```python
from build123d import *

# Parameters (mm, degrees)
BOSS_EXTRUDE1_DEPTH = 4
SKETCH7_R           = 2
CUT_EXTRUDE1_DEPTH  = 4


with BuildPart() as part:
    # Sketch1 → Boss-Extrude1 (new body)
    with BuildSketch(Plane(origin=(0, 0, 0), x_dir=(1, 0, 0), z_dir=(0, 1, 0))):
        Polygon((-125, 115), (-125, 65), (-85, 41.905989232), (-85, -41.905989232), (-125, -65), (-125, -115), (-115, -125), (-65, -125), (-41.905989232, -85), (41.905989232, -85), (65, -125), (115, -125), (125, -115), (125, -65), (85, -41.905989232), (85, 41.905989232), (125, 65), (125, 115), (115, 125), (65, 125), (41.905989232, 85), (-41.905989232, 85), (-65, 125), (-115, 125), align=None)
    extrude(amount=BOSS_EXTRUDE1_DEPTH)

    # Sketch7 → Cut-Extrude1 (cut)
    with BuildSketch(Plane.XZ):
        with Locations(Location((96.392180149, -96.396634108, 0), (0, 0, 270))):
            Circle(SKETCH7_R)
        with Locations(Location((-96.396634108, -96.392180149, 0), (0, 0, 270))):
            Circle(SKETCH7_R)
        with Locations(Location((-96.392180149, 96.396634108, 0), (0, 0, 270))):
            Circle(SKETCH7_R)
        with Locations(Location((96.396634108, 96.392180149, 0), (0, 0, 270))):
            Circle(SKETCH7_R)
        with BuildLine():
            Line((112.617319154, -91.199448609), (97.141666667, -78.666998145))
            Line((97.141666667, -78.666998145), (95.253658711, -80.998398145))
            Line((95.253658711, -80.998398145), (110.729311198, -93.530848609))
            ThreePointArc((110.729311198, -93.530848609), (111.462995743, -94.910428371), (110.980579079, -96.396634108))
            ThreePointArc((110.980579079, -96.396634108), (103.942611055, -103.946782572), (96.392180149, -110.984447587))
            ThreePointArc((96.392180149, -110.984447587), (94.905955053, -111.466804606), (93.526404737, -110.733064696))
            Line((93.526404737, -110.733064696), (80.994575353, -95.256909268))
            Line((80.994575353, -95.256909268), (78.663099585, -97.144823658))
            Line((78.663099585, -97.144823658), (91.194928969, -112.620979086))
            ThreePointArc((91.194928969, -112.620979086), (94.643804759, -114.455328861), (98.359367499, -113.249436313))
            ThreePointArc((98.359367499, -113.249436313), (106.063888832, -106.068145481), (113.245488856, -98.363912355))
            ThreePointArc((113.245488856, -98.363912355), (114.451530517, -94.648398013), (112.617319154, -91.199448609))
        make_face()
        with BuildLine():
            Line((-91.199448609, -112.617319154), (-78.666998145, -97.141666667))
            Line((-78.666998145, -97.141666667), (-80.998398145, -95.253658711))
            Line((-80.998398145, -95.253658711), (-93.530848609, -110.729311198))
            ThreePointArc((-93.530848609, -110.729311198), (-94.910428371, -111.462995743), (-96.396634108, -110.980579079))
            ThreePointArc((-96.396634108, -110.980579079), (-103.946782572, -103.942611055), (-110.984447587, -96.392180149))
            ThreePointArc((-110.984447587, -96.392180149), (-111.466804606, -94.905955053), (-110.733064696, -93.526404737))
            Line((-110.733064696, -93.526404737), (-95.256909268, -80.994575353))
            Line((-95.256909268, -80.994575353), (-97.144823658, -78.663099585))
            Line((-97.144823658, -78.663099585), (-112.620979086, -91.194928969))
            ThreePointArc((-112.620979086, -91.194928969), (-114.455328861, -94.643804759), (-113.249436313, -98.359367499))
            ThreePointArc((-113.249436313, -98.359367499), (-106.068145481, -106.063888832), (-98.363912355, -113.245488856))
            ThreePointArc((-98.363912355, -113.245488856), (-94.648398013, -114.451530517), (-91.199448609, -112.617319154))
        make_face()
        with BuildLine():
            Line((-112.617319154, 91.199448609), (-97.141666667, 78.666998145))
            Line((-97.141666667, 78.666998145), (-95.253658711, 80.998398145))
            Line((-95.253658711, 80.998398145), (-110.729311198, 93.530848609))
            ThreePointArc((-110.729311198, 93.530848609), (-111.462995743, 94.910428371), (-110.980579079, 96.396634108))
            ThreePointArc((-110.980579079, 96.396634108), (-103.942611055, 103.946782572), (-96.392180149, 110.984447587))
            ThreePointArc((-96.392180149, 110.984447587), (-94.905955053, 111.466804606), (-93.526404737, 110.733064696))
            Line((-93.526404737, 110.733064696), (-80.994575353, 95.256909268))
            Line((-80.994575353, 95.256909268), (-78.663099585, 97.144823658))
            Line((-78.663099585, 97.144823658), (-91.194928969, 112.620979086))
            ThreePointArc((-91.194928969, 112.620979086), (-94.643804759, 114.455328861), (-98.359367499, 113.249436313))
            ThreePointArc((-98.359367499, 113.249436313), (-106.063888832, 106.068145481), (-113.245488856, 98.363912355))
            ThreePointArc((-113.245488856, 98.363912355), (-114.451530517, 94.648398013), (-112.617319154, 91.199448609))
        make_face()
        with BuildLine():
            Line((91.199448609, 112.617319154), (78.666998145, 97.141666667))
            Line((78.666998145, 97.141666667), (80.998398145, 95.253658711))
            Line((80.998398145, 95.253658711), (93.530848609, 110.729311198))
            ThreePointArc((93.530848609, 110.729311198), (94.910428371, 111.462995743), (96.396634108, 110.980579079))
            ThreePointArc((96.396634108, 110.980579079), (103.946782572, 103.942611055), (110.984447587, 96.392180149))
            ThreePointArc((110.984447587, 96.392180149), (111.466804606, 94.905955053), (110.733064696, 93.526404737))
            Line((110.733064696, 93.526404737), (95.256909268, 80.994575353))
            Line((95.256909268, 80.994575353), (97.144823658, 78.663099585))
            Line((97.144823658, 78.663099585), (112.620979086, 91.194928969))
            ThreePointArc((112.620979086, 91.194928969), (114.455328861, 94.643804759), (113.249436313, 98.359367499))
            ThreePointArc((113.249436313, 98.359367499), (106.068145481, 106.063888832), (98.363912355, 113.245488856))
            ThreePointArc((98.363912355, 113.245488856), (94.648398013, 114.451530517), (91.199448609, 112.617319154))
        make_face()
    extrude(amount=-CUT_EXTRUDE1_DEPTH, mode=Mode.SUBTRACT)


solid = part.part
```
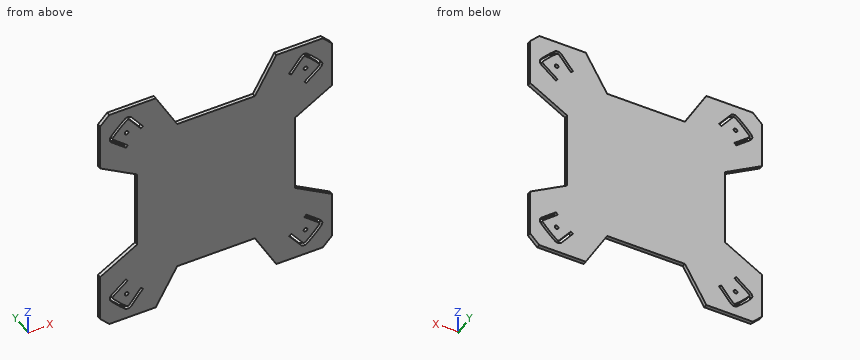
Input: part model. Units: mm. Frame: model coordinates. Give positions to 0.01 mm unless a question says otherwise; leave off trailing zeros. Order: outer loops, then holes, each group sorted by start corner. A loop starts at its lowest first (then second) coordinate and runs counter-clockwise, first axis right, second up. Notation, with made-up numbers: (89, 23.5) - (131, 23.5) arc R18 ccw to (131, 40.5) - close; hole circle Ø2 at (-15.75, 29). An arc over 180 degrees is marked (long way). One line per item, written item: value.
1. Line query: probe 1 along Z at (x, y) = (-91.5, 1.5); probe 2 along Z at (x, y) = (-95, 3.8); probe 3 along X at (y, z) = (2.55, -19). Output: solid intervals per line, ascending.
Determined:
probe 1: -125 to -112.96, -108.22 to -45.66, 45.66 to 108.23, 112.96 to 125
probe 2: -125 to -114.47, -111.47 to -97.82, -94.96 to -47.68, 47.68 to 94.96, 97.83 to 111.47, 114.47 to 125
probe 3: -85 to 85
2. Pin query (flat end, axial travel): pin 1 Ø2 at (x, y) = (-16.5, 2) entering from -Z; pin 2 Ø1 at (y, z) = (2.5, -17) entering from +X; pin 3 Ø3.5 at (x, z) = (96.4, 96.39) entering from +Y; pin 4 Ø1 at (x, y) = (-61, 2) entering from +Z. Return the tip coordinate at first contact, or that it passes through.
Determined:
pin 1: z = -85
pin 2: x = 85
pin 3: through
pin 4: z = 118.94
3. Cut plane A-A, the plane z = -2. Output: boundary loops of the cut face in (x, y), and give its area (3 significant figures).
Determined:
outline: (-85, 0) - (85, 0) - (85, 4) - (-85, 4) - close
area: 680 mm2
4. Cut plane B-B, the plane x = -25. Output: boundary loops of the cut face in (y, z).
Determined:
outline: (0, -85) - (4, -85) - (4, 85) - (0, 85) - close
5. Cut plane C-C, the plane y = 2.45. Give the number of separate pieces and of enclosed holes in the cut face, and give its area (3 significant figures).
Determined:
separate pieces: 1
enclosed holes: 8
area: 44,300 mm2
